from build123d import *

# Parameters (mm, degrees)
F1_DEPTH = 901.7


# Not quite as in the source:
# - a feature names something its author has since deleted; it is built from what else it names


with BuildPart() as f1:
    # F0 (on Top) → F1 (new body)
    with BuildSketch(Plane.XY):
        with BuildLine():
            ThreePointArc((-297.3647676133, -1105.7196050937), (-380.9510446566, -968.4252745053), (-400.480099263, -808.8789961161))
            Line((-400.480099263, -808.8789961161), (-455.3190686334, -1411.5741151153))
            ThreePointArc((-455.3190686334, -1411.5741151153), (-406.2265189052, -1243.2133743356), (-297.3647676132, -1105.7196050937))
        make_face()
        with BuildLine():
            ThreePointArc((-297.3647676133, -1105.7196050937), (-7.9006621425, -1224.1765088207), (272.7039865955, -1086.0369507529))
            ThreePointArc((272.7039865955, -1086.0369507529), (-15.7762559112, -996.0756718787), (-297.3647676132, -1105.7196050937))
        make_face()
        with BuildLine():
            ThreePointArc((355.1002524449, -782.7912184935), (358.7374692929, -813.000356121), (359.9524579315, -843.4034011198))
            ThreePointArc((359.9524579315, -843.4034011198), (337.477444802, -972.3252138184), (272.7039865955, -1086.0369507529))
            ThreePointArc((272.7039865955, -1086.0369507529), (390.7896356908, -1215.6949507084), (451.377353416, -1380.2687819682))
            Line((451.377353416, -1380.2687819682), (355.1002524449, -782.7912184935))
        make_face()
        with BuildLine():
            ThreePointArc((451.377353416, -1380.2687819682), (390.7896356908, -1215.6949507084), (272.7039865955, -1086.0369507529))
            ThreePointArc((272.7039865955, -1086.0369507529), (-7.9006621425, -1224.1765088207), (-297.3647676133, -1105.7196050937))
            ThreePointArc((-297.3647676132, -1105.7196050937), (-406.2265189052, -1243.2133743356), (-455.3190686334, -1411.5741151153))
            ThreePointArc((-455.3190686334, -1411.5741151153), (-20.7359810574, -1909.7329262105), (457.2, -1453.0034011198))
            ThreePointArc((457.2, -1453.0034011198), (455.7420136337, -1416.5197471212), (451.377353416, -1380.2687819682))
        make_face()
    extrude(amount=F1_DEPTH)


solid = f1.part
Input: part model. Units: mm. Frame: model coordinates. Coordinates: 2 decimals unless noted, no trailing zeros. Loops run counter-clockwise (first coordinate to the right, second up) from the corner with the lowest first, then second, coordinate; pieces in that order, holes last. Notation, with made-up numbers: (62, 35) - (95, 35) arc R22 cw to (95, 71) - close; hole circle Ø5 at (22, 26.25). An arc over 180 degrees is marked (long way). Answer in a Markdown table with one row per item. Add a question column.
Item 1: Mould query, pull axis X, two halves, no side actions, for faces 1 (the cylindrical face through (4.923, -1910.177, 444.538)), 2 (the flat face through (-6, -1464, 901.7)), 3 (the cylindrical face through (-380.201, -970.565, 444.538)). Classes: released by +X, released by -X, zero draft, split by the parting line, or undercut.
Item 2: Section query D-D on y = -1202. Return the cut outline in (x, z).
Item 3: Line query: line 1 along X through (y, z) = (-936, 81); line 2 along X through (y, z) = (-1066.5, 83); line 3 along X through (y, z) = (-902, 510). Output: solid intervals per line, ascending. Write a range as [from, to].
Item 4: Section query A-A on z = 810. Return the cut outline in (x, y), then the cut area to 3 significant figures.
Item 5: Contact query for flat-ended pins moving along their axis: P1, Ø6, axis at y = -1706, z = 684.5, coming from the -X side; P2, Ø1, axis at y = -1118, z = 747, coming from the +X side; P3, Ø2, axis at x = 175.5, z = 703.5, coming from the +Y side; P4, Ø10, axis at x = 318.5, y = -1561.5, coming from the -Z side. Output: stop coordinate, or through.
Item 6: Section query B-B on y = -1057. Return the cut outline in (x, z), then the cut area to 3 significant figures.
Item 7: Section query C-C on x = 0. Return the cut outline in (y, z), then the cut area to 3 significant figures.
Recorded:
| question | item | result |
|---|---|---|
| 1 | face 1 | split by the parting line |
| 1 | face 2 | zero draft |
| 1 | face 3 | undercut |
| 2 | outline | (-436.25, 0) - (422.65, 0) - (422.65, 901.7) - (-436.25, 901.7) - close |
| 3 | line 1 | [-412.05, -390.62], [348.53, 379.79] |
| 3 | line 2 | [-423.92, -329.9], [-244.23, 244.23], [287.8, 400.82] |
| 3 | line 3 | [-408.95, -397.51], [355.42, 374.31] |
| 4 | outline | (-455.32, -1411.57) arc R457.2 ccw (long way) to (451.38, -1380.27) - (355.1, -782.79) arc R381 cw to (272.7, -1086.04) arc R457.2 ccw to (-297.36, -1105.72) arc R381 cw to (-400.48, -808.88) - close |
| 4 | area | 705,000 mm^2 |
| 5 | P1 | x = -382.8 |
| 5 | P2 | x = 409.2 |
| 5 | P3 | y = -1030.41 |
| 5 | P4 | z = 0 |
| 6 | outline | (-423.06, 0) - (-336.54, 0) - (-336.54, 901.7) - (-423.06, 901.7) - close; (-228.5, 0) - (228.5, 0) - (228.5, 901.7) - (-228.5, 901.7) - close; (294.45, 0) - (399.29, 0) - (399.29, 901.7) - (294.45, 901.7) - close |
| 6 | area | 585,000 mm^2 |
| 7 | outline | (-1910.2, 0) - (-995.8, 0) - (-995.8, 901.7) - (-1910.2, 901.7) - close |
| 7 | area | 825,000 mm^2 |
